from build123d import *

# Parameters (mm, degrees)
SKETCH1_W             = 15
SKETCH1_H             = 15
BOSS_EXTRUDE1_DEPTH   = 57.15
M5X0_8_TAPPED_HOLE1_D = 4.2
M5X0_8_TAPPED_HOLE2_D = 4.2
SKETCH12_W            = 30
SKETCH12_H            = 8.246203466
CUT_EXTRUDE2_DEPTH    = 1.53
FILLET2_R             = 3.175


with BuildPart() as part:
    # Sketch1 → Boss-Extrude1 (new body)
    with BuildSketch(Plane(origin=(0, 0, 0), x_dir=(0, 0, -1), z_dir=(1, 0, 0))):
        Rectangle(SKETCH1_W, SKETCH1_H)
    extrude(amount=BOSS_EXTRUDE1_DEPTH)

    # M5x0.8 Tapped Hole1 (through all)
    with Locations(Plane.XY.offset(7.5)):
        with Locations((5, 0), (52.15, 0)):
            Hole(M5X0_8_TAPPED_HOLE1_D / 2)

    # M5x0.8 Tapped Hole2 (through all)
    with Locations(Plane(origin=(0, -7.5, 0), x_dir=(-1, 0, 0), z_dir=(0, -1, 0))):
        with Locations((-5, 0), (-52.15, 0)):
            Hole(M5X0_8_TAPPED_HOLE2_D / 2)

    # Sketch12 → Cut-Extrude2 (cut)
    with BuildSketch(Plane.XY.offset(7.5)):
        with Locations((28.575, -7.5)):
            Rectangle(SKETCH12_W, SKETCH12_H)
    extrude(amount=-CUT_EXTRUDE2_DEPTH, mode=Mode.SUBTRACT)

    # Fillet2
    fillet2_edges = [part.edges().sort_by_distance(p)[0] for p in [
        (43.575, -3.376898267, 6.735),
        (13.575, -3.376898267, 6.735),
    ]]
    fillet(fillet2_edges, radius=FILLET2_R)


solid = part.part
Geometry: final body of the model. Coordinates: model frame, mm. A direction names the side the tool comes from. Round coordinates to 2 decimals unless told otherwise and drop trailing zeros. Loops run counter-clockwise (first coordinate to the right, second up) from the corner with the lowest first, then second, coordinate; pieces in that order, holes last.
Q1. Section B-B on z = 1.5. Return loops of the section in (x, y).
Q2. Section D-D on x = 17.5. Return loops of the section in (y, z), plus the area to 3 significant figures.
Q3. Pin query (flat end, axial travel): P1, Ø0.5, axis at x = 32.5, z = 6.5, coming from the -Y side; P2, Ø1.2, axis at x = 27, y = -6, coming from the +Z side. Return the tip coordinate at first contact, or that it passes through.
Q4. Material intervals for L1, parallel to X at y = 0, z = -2.5; L2, parallel to Y at x = 52.15, z = -4; L3, parallel to X at y = -2.75, z = -1.75, sorted ascending.
Q5. Section A-A on x = 52.15. Return loops of the section in (y, z), plus the area to 3 significant figures.
Q6. Section C-C on y = 4.5. Return loops of the section in (x, z).
Q7. Pull-direction query (Z, two-part tool) for faces 1 (the flat face through (28, 0, -7.5)), 2 (the cylindrical face through (2.997, 0.631, 4.531)), 3 (the cylindrical face through (50.5, 4.6, 1.3)); classes: released by +Z, released by -Z, zero draft, split by the parting line, or undercut.
Q8. Access query for faces 4 (the cylindrical face through (14.53, -4.28, 6.72)), 5 (the cylindrical face through (53.8, -1.3, -4.6)). Directions: +Z, -Z, +X, -X, +Y, -Y. A direction counts if a zero-diameter tool reaches every point of the face in a straight line with its end or side. Return the directions, or none.
Evaluation:
1. outline: (0, -7.5) - (3.53, -7.5) - (3.53, -1.5) arc R2.1 cw to (3.53, 1.5) - (3.53, 7.5) - (0, 7.5) - close; (6.47, -7.5) - (50.68, -7.5) - (50.68, -1.5) arc R2.1 cw to (50.68, 1.5) - (50.68, 7.5) - (6.47, 7.5) - (6.47, 1.5) arc R2.1 cw to (6.47, -1.5) - close; (53.62, -7.5) - (57.15, -7.5) - (57.15, 7.5) - (53.62, 7.5) - (53.62, 1.5) arc R2.1 cw to (53.62, -1.5) - close
2. outline: (-7.5, -7.5) - (7.5, -7.5) - (7.5, 7.5) - (-3.38, 7.5) - (-3.38, 5.97) - (-7.5, 5.97) - close
2. area: 219 mm2
3. P1: stops at y = -3.38
3. P2: stops at z = 5.97
4. L1: x = 0 to 2.9, 7.1 to 50.05, 54.25 to 57.15
4. L2: y = -7.5 to -2.1, 2.1 to 7.5
4. L3: x = 0 to 3.84, 6.16 to 50.99, 53.31 to 57.15
5. outline: (-7.5, -7.5) - (-2.1, -7.5) - (-2.1, -2.1) - (-7.5, -2.1) - close; (-7.5, 2.1) - (-2.1, 2.1) - (-2.1, 7.5) - (-7.5, 7.5) - close; (2.1, -7.5) - (7.5, -7.5) - (7.5, -2.1) - (2.1, -2.1) - close; (2.1, 2.1) - (7.5, 2.1) - (7.5, 7.5) - (2.1, 7.5) - close
5. area: 117 mm2
6. outline: (0, -7.5) - (57.15, -7.5) - (57.15, 7.5) - (0, 7.5) - close; hole circle Ø4.2 at (5, 0); hole circle Ø4.2 at (52.15, 0)
7. face 1: released by -Z
7. face 2: zero draft
7. face 3: undercut
8. face 4: +Z, -Y
8. face 5: +Z, -Z
